```python
from build123d import *

# Parameters (mm, degrees)
SKETCH1_W           = 108
SKETCH1_H           = 54
SKETCH1_R           = 4
BOSS_EXTRUDE3_DEPTH = 11
BOSS_EXTRUDE4_DEPTH = 26
CUT_EXTRUDE1_START  = -21
CUT_EXTRUDE1_DEPTH  = 43.68843134
FILLET1_R           = 10


# Read off the part's stored shape, not the designer's step: Cut-Extrude1
with BuildPart() as part:
    # Sketch1 → Boss-Extrude3 (new body)
    with BuildSketch(Plane(origin=(0, 0, 0), x_dir=(1, 0, 0), z_dir=(0, 1, 0))):
        Rectangle(SKETCH1_W, SKETCH1_H)
        with Locations(Location((-44, -8, 0), (0, 0, 270))):
            Circle(SKETCH1_R, mode=Mode.SUBTRACT)
        with Locations(Location((-44, 17, 0), (0, 0, 270))):
            Circle(SKETCH1_R, mode=Mode.SUBTRACT)
        with Locations(Location((44, 17, 0), (0, 0, 90))):
            Circle(SKETCH1_R, mode=Mode.SUBTRACT)
        with Locations(Location((44, -8, 0), (0, 0, 90))):
            Circle(SKETCH1_R, mode=Mode.SUBTRACT)
    extrude(amount=BOSS_EXTRUDE3_DEPTH)

    # Sketch4 → Boss-Extrude4 (add, symmetric)
    with BuildSketch(Plane(origin=(0, 0, 0), x_dir=(0, 0, -1), z_dir=(1, 0, 0))):
        with BuildLine():
            Line((9.945906404, 32), (9.945906404, 23))
            Line((9.945906404, 23), (21, 23))
            Line((21, 23), (21, 11))
            Line((21, 11), (-27, 11))
            ThreePointArc((-27, 11), (-11.302622957, 26.383151285), (9.945906404, 32))
        make_face()
    extrude(amount=BOSS_EXTRUDE4_DEPTH, both=True)

    # Cut-Extrude1 outline → Cut-Extrude1 (cut)
    with BuildSketch(Plane.XY.offset(CUT_EXTRUDE1_START)):
        Polygon((-9, 17), (9, 17), (17, 32), (-17, 32), align=None)
    extrude(amount=CUT_EXTRUDE1_DEPTH, mode=Mode.SUBTRACT)

    # Fillet1
    fillet1_edges = [part.edges().sort_by_distance(p)[0] for p in [
        (54, 5.5, 27),
        (-54, 5.5, 27),
    ]]
    fillet(fillet1_edges, radius=FILLET1_R)


solid = part.part
```
Geometry check sheet. Reference: the model listing, model coordinates, mm. A direction names the side the tool comes from. Coordinates: 2 decimals unless noted, no trailing zeros. Order: outer loops, then holes, each group sorted by start corner. A loop starts at its lowest first (then second) coordinate and runs counter-clockwise, first axis right, second up. Notation, with made-up numbers: (45, 16.5) - (54, 16.5) arc R16 ccw to (54, 29.5) - close; hole circle Ø7 at (-11.5, 15). An arc over 180 degrees is marked (long way). Answer as a JSON object with one key per item and string values. Group by question number.
Item 1: Scan lines: probe 1 along X at (y, z) = (6, -17); probe 2 along Z at (x, y) = (44, 7); probe 3 along Z at (x, y) = (-41, 9). Record each from-to range of solid material in increasing order.
Item 2: Draft check along X on faces 5 (the face through (-21, 28, -9.946)), 6 (the face through (-40.034, 5.423, -17.521)), 7 (the face through (-54, 5, -5)). Enter one of: +X half, -X half, draft (parallel to the pull), parting line (faces both ways), or undercut.
Item 3: Sectioned sample at B-B, the plane x = -4. Record the cut outline in (y, z).
Item 4: Sectioned sample at A-A, the plane z = -17. Record the cut outline in (x, y).
Item 5: Tool access check on faces 1 (the face through (-26, 19, 3)), 2 (the face through (12.055, 22.728, 0.538)), 3 (the face through (50.99, 5.58, 24.15)), 4 (the face through (-19, 23, -15)). Record the directions out of +Z, -Z, +X, -X, +Y, -Y that give a thin tool (end or side, any length) a straight path to the whole face; none if there is none.
Item 6: Depth check by flat-ended pin: pin 1 Ø17 at (y, z) = (24, 10.5) entering from +X; pin 2 Ø4.5 at (x, y) = (-19.5, 26) entering from -Z; pin 3 Ø3.5 at (x, z) = (-22.5, -17) entering from +Y. Enter the tip coordinate at first touch or a pass-through.
Item 7: Sectioned sample at C-C, the plane y = 9.5. Record the cut outline in (x, z), and give its area (3 significant figures).
Item 8: Sectioned sample at D-D, the plane x = 23. Record the cut outline in (y, z), and give its area (3 significant figures).
Resolved:
{
 "1": {"probe 1": "-54 to -48, -40 to 40, 48 to 54", "probe 2": "-27 to -21, -13 to 4, 12 to 27", "probe 3": "-27 to -19.65, -14.35 to 5.35, 10.65 to 27"},
 "2": {"face 5": "draft", "face 6": "undercut", "face 7": "-X half"},
 "3": {"outline": "(0, -27) - (11, -27) - (11, -21) - (17, -21) - (17, 22.69) arc R43 ccw to (11, 27) - (0, 27) - close"},
 "4": {"outline": "(-54, 0) - (-48, 0) - (-48, 11) - (-54, 11) - close; (-40, 0) - (40, 0) - (40, 11) - (26, 11) - (26, 23) - (12.2, 23) - (9, 17) - (-9, 17) - (-12.2, 23) - (-26, 23) - (-26, 11) - (-40, 11) - close; (48, 0) - (54, 0) - (54, 11) - (48, 11) - close"},
 "5": {"face 1": "+Z, -Z, -X, +Y", "face 2": "+Z, -Z, +Y", "face 3": "+Z, +X, +Y, -Y", "face 4": "-Z, +X, -X, +Y"},
 "6": {"pin 1": "x = 26", "pin 2": "z = -9.95", "pin 3": "y = 23"},
 "7": {"outline": "(-54, -27) - (54, -27) - (54, 17) arc R10 ccw to (44, 27) - (-44, 27) arc R10 ccw to (-54, 17) - close; hole circle Ø8 at (-44, -17); hole circle Ø8 at (-44, 8); hole circle Ø8 at (44, -17); hole circle Ø8 at (44, 8)", "area": "5,590 mm^2"},
 "8": {"outline": "(0, -27) - (11, -27) - (11, -21) - (23, -21) - (23, -9.95) - (32, -9.95) arc R43 ccw to (11, 27) - (0, 27) - close", "area": "1,280 mm^2"}
}
